```python
from build123d import *

# Parameters (mm, degrees)
F2_T = -2.54
F4_D = 48.26


with BuildPart() as f1:
    # F0 (on Front) → F1 (revolve)
    with BuildSketch(Plane.XZ):
        Polygon((-115.680311, 25.4), (-115.680311, 0), (290.719689, 0), (290.719689, 25.4), (278.019689, 25.4), (239.919689, 50.8), (-64.880311, 50.8), (-102.980311, 25.4), align=None)
    revolve(axis=Axis((87.519689, 0, 0), (-1, 0, 0)))

    # F2
    f2_openings = [f1.faces().sort_by_distance(p)[0] for p in [
        (-115.680311, 0, 0),
    ]]
    offset(amount=F2_T, openings=f2_openings)

    # F4 (through all)
    with Locations(Plane.YZ.offset(290.719689)):
        with Locations((0, 0)):
            Hole(F4_D / 2)


solid = f1.part
```
Work out the finished part from the listing and answer in its coordinate system (mm). A direction names the side the tool comes from. Coordinates: 2 decimals unless noted, no trailing zeros. Loops run counter-clockwise (first coordinate to the right, second up) from the corner with the lowest first, then second, coordinate; pieces in that order, holes last. Notation, with made-up numbers: M 36.5,0.5 L 64.5,0.5 A20 ccw 64.5,20.5 Z; hole C 43,82.25 d10. An arc over 180 degrees is marked long. Use CSV: the item, a comma, the result in double quotes. Start each with the question number.
(1) Consider line 1 (Y direction, x = -105, z = 0); line 2 (Y direction, x = -37.5, z = -2.5); line 3 (X direction, y = -37.5, z = -15.5) (3 decimals). Determine where each line is inside the solid, lowest interval first.
(2) Given pin 1 Ø3 at (y, z) = (28.5, 29.5) entering from +X; pin 2 Ø4 at (x, z) = (158.5, -23) entering from -Y; pin 3 Ø10 at (x, z) = (-67.5, 24.5) entering from +Y, each flat-ended and moving along its own axis, determine where each tip first touches the part or whether it passes through.
(3) For faces 1 (the face through (284.281, -24.796, -5.506)), 2 (the face through (282.93, -12.97, 20.35)), 3 (the face through (85.4, 47.85, -6.28)), determine the directions among +Z, -Z, +X, -X, +Y, -Y from which every point of the face is accessible in a straight line to the end or side of a thin tool.
(4) Find section D-D, the plane x = -82. Give the vertices of the cut face in (y, z).
(5) Find section A-A, the plane z = 0. Give the vertices of the cut face in (x, y).
(6) For a pull along Y with two mould halves and no side action, classify faces 4 (the face through (290.72, -9.3, -22.5)), 5 (the face through (-109.419, -24.796, -5.506)), 6 (the face through (-108.1, -12.97, 20.35)) as +Y half, -Y half, draft (parallel to the pull), parting line (faces both ways), or undercut.
(7) Find section C-C, the plane x = 178.5. Give the vertices of the cut face in (y, z), then the cut area to 3 significant figures.
Recorded:
1,line 1,"y = -25.4 to -24.13, 24.13 to 25.4"
1,line 2,"y = -50.74 to -48.2, 48.2 to 50.74"
1,line 3,"x = -80.215 to -75.636, 250.675 to 255.254"
2,pin 1,"stops at x = 256.84"
2,pin 2,"stops at y = -46.26"
2,pin 3,"stops at y = 46.59"
3,face 1,"+X"
3,face 2,"+X, -X"
3,face 3,"none"
4,outline,"C 0,0 d78.77; hole C 0,0 d72.67"
5,outline,"M -115.68,-25.4 L -102.98,-25.4 L -64.88,-50.8 L 239.92,-50.8 L 278.02,-25.4 L 290.72,-25.4 L 290.72,-24.13 L 275.35,-24.13 L 239.15,-48.26 L -64.11,-48.26 L -100.31,-24.13 L -115.68,-24.13 Z; M -115.68,24.13 L -100.31,24.13 L -64.11,48.26 L 239.15,48.26 L 275.35,24.13 L 290.72,24.13 L 290.72,25.4 L 278.02,25.4 L 239.92,50.8 L -64.88,50.8 L -102.98,25.4 L -115.68,25.4 Z"
6,face 4,"draft"
6,face 5,"parting line"
6,face 6,"undercut"
7,outline,"C 0,0 d101.6; hole C 0,0 d96.52"
7,area,"790 mm^2"
